Design review of the part built by this model. Coordinates are the model's own, in mm. A direction names the side the tool comes from. Round coordinates to 2 decimals unless told otherwise and drop trailing zeros. Order: outer loops, then holes, each group sorted by start corner. A loop starts at its lowest first (then second) coordinate and runs counter-clockwise, first axis right, second up. Notation, with made-up numbers: (33, -10) - (62, -10) arc R27 ccw to (62, 22) - close; hole circle Ø8 at (28.25, -35.75). An arc over 180 degrees is marked (long way). Write item = value, one per line.
from build123d import *

# Parameters (mm, degrees)
ESQUISSE1_R                  = 6.5
BOSS_EXTRU_1_DEPTH           = 147
ESQUISSE2_R                  = 3.5
BOSS_EXTRU_2_DEPTH           = 50
CONG_1_R                     = 3
CHANFREIN1_SIZE              = 16
CHANFREIN1_SIZE2             = 2.821231691
ENL_V_MAT_EXTRU_1_DEPTH      = 198.214350391
ENL_V_MAT_EXTRU_1_DEPTH_BACK = 198.214350391
ENL_V_MAT_EXTRU_2_DEPTH      = 5


with BuildPart() as part:
    # Esquisse1 → Boss.-Extru.1 (new body)
    with BuildSketch(Plane.XY):
        Circle(ESQUISSE1_R)
    extrude(amount=BOSS_EXTRU_1_DEPTH)

    # Esquisse2 → Boss.-Extru.2 (add)
    with BuildSketch(Plane.XY.offset(147)):
        Circle(ESQUISSE2_R)
    extrude(amount=BOSS_EXTRU_2_DEPTH)

    # Congé1
    cong_1_edges = [part.edges().sort_by_distance(p)[0] for p in [
        (-3.5, 0, 197),
    ]]
    fillet(cong_1_edges, radius=CONG_1_R)

    # Chanfrein1
    chanfrein1_edges = [part.edges().sort_by_distance(p)[0] for p in [
        (-6.5, 0, 147),
    ]]
    chanfrein1_side = [part.faces().sort_by_distance(p)[0] for p in [
        (-6.5, 0, 73.5),
    ]]
    chamfer(chanfrein1_edges, length=CHANFREIN1_SIZE, length2=CHANFREIN1_SIZE2, reference=chanfrein1_side[0])

    # Esquisse3 → Enlèv. mat.-Extru.1 (cut, two sides: drawn at the far end of the back side and taken through both)
    with BuildSketch(Plane(origin=(0, 0, 0), x_dir=(1, 0, 0), z_dir=(0, 1, 0)).offset(-ENL_V_MAT_EXTRU_1_DEPTH_BACK)):
        Polygon((6.5, 0), (-6.5, -1.827030851), (-6.5, 0), align=None)
    extrude(amount=ENL_V_MAT_EXTRU_1_DEPTH + ENL_V_MAT_EXTRU_1_DEPTH_BACK, mode=Mode.SUBTRACT)

    # Esquisse4 → Enlèv. mat.-Extru.2 (cut)
    with BuildSketch(Plane(origin=(0.125899488, 0, 0.895821406), x_dir=(-0.9902680687415714, 0, 0.1391731009600587), z_dir=(-0.1391731009600587, 0, -0.9902680687415714))):
        with BuildLine():
            Line((-1.607582844, 1.189822423), (-1.607582844, -1.189822423))
            ThreePointArc((-1.607582844, -1.189822423), (2, 0), (-1.607582844, 1.189822423))
        make_face()
    extrude(amount=-ENL_V_MAT_EXTRU_2_DEPTH, mode=Mode.SUBTRACT)


solid = part.part
Item 1: For faces 1 (the face through (3.233, -1.341, 170.171)), 2 (the face through (-5.158, -3.955, 64.583)), list the 3-axis set-ups (+Z, -Z, +X, -X, +Y, -Y) from which the entire face can be reached by the end or side of a thin tool; tool diameter is ignored.
Data:
face_1 = +Z
face_2 = +Z, -Z
Item 2: The part is to be moulded in two halves that separate along Y. For faces 3 (the face through (4.836, 1.523, 139.112)), 4 (the face through (-1.51, -0.07, 3.62)), 5 (the face through (-2.798, -0.091, 1.307)), 6 (the face through (0.65, 0.03, 5.87)), say which applies: +Y half, -Y half, draft (parallel to the pull), parting line (faces both ways), or undercut.
Data:
face_3 = parting line
face_4 = undercut
face_5 = draft
face_6 = undercut
Item 3: For line 1 along Y through (x, z) = (0.25, 12); line 2 along X through (y, z) = (0.25, 150); line 3 along X through (y, z) = (0.5, 124.5), list the stretches that pass through material, from the lowest coordinate up. Write a range as [from, to].
Data:
line_1 = [-6.5, 6.5]
line_2 = [-3.49, 3.49]
line_3 = [-6.48, 6.48]
Item 4: Insertion check: P1, Ø4, axis at x = -1.5, y = 2.5, coming from the +Z side; P2, Ø4, axis at x = -2, z = 140, coming from the +Y side; P3, Ø1, axis at y = 1, z = 62.5, coming from the +X side. Each pin has a flat end and moves straight along its axis. Give the tip position at first contact, or say it passes through.
Data:
P1 = 196.97
P2 = 5.13
P3 = 6.48
Item 5: Take a section at A-A, the plane z = 46.5. State the section outline as (x, y) points.
Data:
outline = circle Ø13 at (0, 0)
Item 6: Take a section at B-B, the plane z = 138.5. State the section outline as (x, y) points, and give its area (3 significant figures).
Data:
outline = circle Ø10.36 at (0, 0)
area = 84.2 mm2
